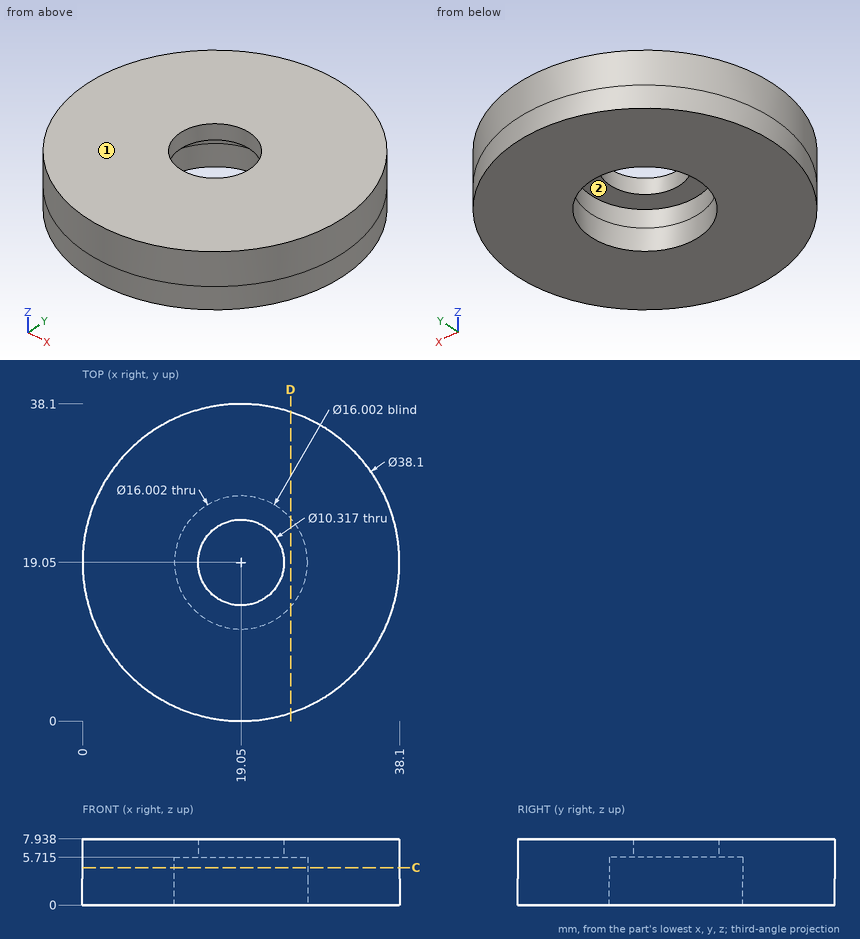
The figure shows three views and two pictorial views of one solid part (mm, origin at its lowest corner). Answer the questions. Round coordinates to 2 decimals unless told otherwise and drop trailing zeros. Loops run counter-clockwise (first coordinate to the right, second up) from the corner with the lowest first, then second, coordinate; pieces in that order, holes last. Notation, with made-up numbers: M 15.5,71 L 54.5,71 A35 ccw 54.5,103 Z; hole C 30,85 d3. An arc over 180 degrees is marked long. Return JSON: item names as keys, results as strings.
Q1. Each of these flat-tipped pins is pushed along its axis until it touches: pin 1 Ø2 at (x, z) = (23.5, 1.5) entering from -Y (1 decimal); pin 2 Ø8.5 at (x, y) = (19.05, 19.05) entering from -Z. Where does it stop, or does it pass through?
Results list:
{"pin 1": "stops at y = 0.3", "pin 2": "passes through"}
Q2. Find section D-D, the plane x = 25. Determine the outline of the cut face in (y, z) (1 decimal), plus the area to 3 significant figures.
Results list:
{"outline": "M 1,0 L 13.7,0 L 13.7,5.7 L 24.4,5.7 L 24.4,0 L 37.1,0 L 37.1,7.9 L 1,7.9 Z", "area": "226 mm2"}
Q3. The mould has two halves that part along Y. Classify the marked faces 1 and 2: released by +Y, released by -Y, zero draft, split by the parting line, or undercut.
Results list:
{"face 1": "zero draft", "face 2": "undercut"}
Q4. Find the intervals of material crossed by line 1 along Y through (x, z) = (19.05, 4.2); line 2 along Z through (x, y) = (17.5, 26) (1 decimal); line 3 along X through (y, z) = (21, 4.5), in increasing order. Write a range as from..to.
Results list:
{"line 1": "y = 0..11.05, 27.05..38.1", "line 2": "z = 5.7..7.9", "line 3": "x = 0.1..11.29, 26.81..38"}
Q5. Find section C-C, the plane z = 4.5. Determine the outline of the cut face in (x, y).
Results list:
{"outline": "C 19.05,19.05 d38.1; hole C 19.05,19.05 d16"}
